Build history of the part. All positions in model axes, mm. A direction names the side the tool comes from. Give positions to 0.01 mm unless a question says otherwise; leave off trailing zeros. Loops run counter-clockwise (first coordinate to the right, second up) from the corner with the lowest first, then second, coordinate; pieces in that order, holes last. Notation, with made-up numbers: M -22,24 L -6,24 A18 ccw -6,56 Z; hole C 7,35.25 d2. An arc over 180 degrees is marked long. Put each result on its own line as item: value.
Autodesk Inventor part; units mm, degrees
ref_plane "Work Plane1" through (0, 0, 0) normal (-0.5, -0.866, 0) x (0, 0, 1)
ref_plane "YZ Plane" through (0, 0, 0) normal (1, 0, 0) x (0, 1, 0)
ref_plane "XY Plane" through (0, 0, 0) normal (0, 0, 1) x (1, 0, 0)
sketch "Sketch1" plane through (0, 0, 0) normal (0, 0, 1) x (1, 0, 0)
  circle A0 centre (0, 0) radius 11.5
  circle A1 centre (0, 0) radius 4
  point P0 (8, 0)
  point P1 (-4, 6.9282)
  point P2 (-4, -6.9282)
  dimension "d0" = 23
  dimension "d1" = 8
  dimension "d2" = 8
  dimension "d5" = 360
extrude "Plate1" add sketch "Sketch1" along normal blind 10
hole "Hole1" at (8, 0, 0) at (-4, 6.9282, 0) at (-4, -6.9282, 0) direction (0, 0, 1) diameter 3.242 depth 15 tip angle 118
sketch "Sketch2" plane through (0, 0, 0) normal (1, 0, 0) x (0, 1, 0)
  line L0 (4, 0) -> (-4, 0)
  point P0 (0, 0)
  point P1 (0, 5)
  dimension "d15" = 5
hole "Hole2" at (0, 0, 5) direction (-1, 0, 0) diameter 2.459 end through all
ref_plane "Work Plane1" through (0, 0, 0) normal (-0.5, -0.866, 0) x (0, 0, 1)
sketch "Sketch3" plane through (0, 0, 0) normal (-0.5, -0.866, 0) x (0, 0, 1)
  point P0 (0, 0)
  point P1 (5, 3.9111)
  point P2 (5, 0)
  dimension "d24" = 5
hole "Hole3" at (0, 0, 5) direction (0.5, 0.866, 0) diameter 2.459 end through all
equation "\"d7\" = Thickness"
equation "\"BendReliefDepth\" = 0.5 * Thickness"
properties part number "as mount 10 mm (3x)" material "Aluminum 6061"
Q1. Slice it at D-D (y = -2.5). List the corners of the cut face in (x, z), and give its area (3 significant figures).
Here are the results:
outline: M -11.22,0 L -3.12,0 L -3.12,10 L -11.22,10 Z; M 3.12,0 L 11.22,0 L 11.22,10 L 3.12,10 Z
area: 162 mm²
Q2. Mould opens along X. For faces 3 (the cylindrical face through (6.18, -9.7, 4.93)), 4 (the flat face through (5, 0, 10)), 5 (the cylindrical face through (-2.562, 7.676, 5.07)) say: pulls with the +X half, pulls with the -X half, needs draft (parallel to the pull), parting line crosses it, or undercut.
Here are the results:
face 3: parting line crosses it
face 4: needs draft
face 5: undercut
Q3. Tool access for faces 1 (the cylindrical face through (4.261, 6.439, 3.864)), 2 (the cylindrical face through (-7.71, -0.05, 6.23)): list every direction of +Z, -Z, +X, -X, +Y, -Y with a clear straight run to the whole face (end or side of a thin tool).
Here are the results:
face 1: none
face 2: -X
Q4. Probe line 1 (X direction, y = 0, z = 5.25); line 2 (Y direction, x = 0, z = 5.75); line 3 (Y direction, x = -10, z = 5.5). List the from-to ranges inside material, lowest first. Write a range as from..to.
Here are the results:
line 1: 4..6.38, 9.62..11.5
line 2: -11.5..-4, 4..11.5
line 3: -5.68..-1.12, 1.12..5.68
Q5. Slice it at A-A (z = 5). List the corners of the cut face in (x, y), and give its area (3 significant figures).
Here are the results:
outline: M -11.43,-1.23 A11.5 ccw long 6.78,9.29 L 2.97,2.68 A4 cw long -3.81,-1.23 Z; M -11.43,1.23 L -3.81,1.23 A4 cw 0.84,3.91 L 4.65,10.52 A11.5 ccw Z; hole C -4,-6.93 d3.24; hole C -4,6.93 d3.24; hole C 8,0 d3.24
area: 303 mm²
Q6. Slice it at C-C (y = 0). List the corners of the cut face in (x, z).
Here are the results:
outline: M -11.5,0 L -4,0 L -4,3.77 L -11.5,3.77 Z; M -11.5,6.23 L -4,6.23 L -4,10 L -11.5,10 Z; M 4,0 L 6.38,0 L 6.38,10 L 4,10 Z; M 9.62,0 L 11.5,0 L 11.5,10 L 9.62,10 Z
Q7. Slice it at B-B (x = 8). List the corners of the cut face in (y, z).
Here are the results:
outline: M -8.26,0 L -1.62,0 L -1.62,10 L -8.26,10 Z; M 1.62,0 L 8.26,0 L 8.26,10 L 1.62,10 Z
Q8. Drop flat-ended pins along their axis: pin 1 Ø2 at (x, z) = (6, 1.5) entering from +Y; pin 2 Ø5 at (y, z) = (-7, 5.5) entering from +X; pin 3 Ø1.5 at (y, z) = (8, 4) entering from +X. Give the stop position or say it passes through.
Here are the results:
pin 1: y = 10.36
pin 2: x = 10.58
pin 3: x = 8.93
